from build123d import *

# Parameters (mm, degrees)
BOSS_EXTRUDE1_DEPTH = 2.54
SKETCH2_R           = 1.016
CUT_EXTRUDE1_DEPTH  = 3.54


with BuildPart() as part:
    # Sketch1 → Boss-Extrude1 (new body)
    with BuildSketch(Plane(origin=(0, 0, 0), x_dir=(1, 0, 0), z_dir=(0, 1, 0))):
        with BuildLine():
            Line((0, 0), (10.16, 0))
            ThreePointArc((10.16, 0), (13.97, 3.81), (10.16, 7.62))
            Line((10.16, 7.62), (0, 7.62))
            ThreePointArc((0, 7.62), (-3.81, 3.81), (0, 0))
        make_face()
    extrude(amount=BOSS_EXTRUDE1_DEPTH)

    # Sketch2 → Cut-Extrude1 (cut, through all)
    with BuildSketch(Plane(origin=(0, 2.54, 0), x_dir=(1, 0, 0), z_dir=(0, 1, 0))):
        with Locations((0, 3.81)):
            Circle(SKETCH2_R)
        with Locations((5.08, 3.81)):
            Circle(SKETCH2_R)
        with Locations((10.16, 3.81)):
            Circle(SKETCH2_R)
    extrude(amount=-CUT_EXTRUDE1_DEPTH, mode=Mode.SUBTRACT)


solid = part.part
Design review of the part built by this model. Coordinates are the model's own, in mm. Round coordinates to 2 decimals unless told otherwise and drop trailing zeros. Loops run counter-clockwise (first coordinate to the right, second up) from the corner with the lowest first, then second, coordinate; pieces in that order, holes last. Notation, with made-up numbers: (-1.75, 79.25) -> (47.25, 79.25) arc R23 cw to (47.25, 112.25) -> close; hole circle Ø4 at (-11.75, -33.75). An arc over 180 degrees is marked (long way). Use one line per item in the form item = value. Start each with the question number.
Q1. For pin 1 Ø1 at (x, y) = (-1, 2) entering from -Z; pin 2 Ø2.5 at (x, z) = (5.08, -3.81) entering from +Y, all flat-tipped, find the tip position at first contact; note any pin that passes through.
Q2. Wall thickness on line 1 along X through (y, z) = (0.55, -3.81); line 2 along Z through (x, y) = (0, 1.6); line 3 along X through (y, z) = (1.45, -4): over which ranges is each line inside the solid? List them lowest first. Write a range as [from, to].
Q3. Draft analysis for pull direction Z (two halves, no side actions). For faces 1 (the face through (-3.81, 1.25, -3.89)), 2 (the face through (-0.132, 1.288, -4.817)), 3 (the face through (7, 0, -4)), 4 (the face through (5, 1, -7.62)), state which applies: +Z half, -Z half, draft (parallel to the pull), parting line (faces both ways), or undercut.
Q4. We need section D-D on z = -2.25. Give the boundary of the cut face in (x, y), then the cut area to 3 significant figures.
Q5. We need section B-B on y = 1.9. Give the boundary of the cut face in (x, z).
Q6. We need section C-C on z = -3.81. Give the boundary of the cut face in (x, y).
Q7. We need section A-A on x = 5.08. Give the boundary of the cut face in (y, z), then the cut area to 3 significant figures.
Calculated:
q1.pin_1 = -7.59
q1.pin_2 = 2.54
q2.line_1 = [-3.81, -1.02], [1.02, 4.06], [6.1, 9.14], [11.18, 13.97]
q2.line_2 = [-7.62, -4.83], [-2.79, 0]
q2.line_3 = [-3.81, -1], [1, 4.08], [6.08, 9.16], [11.16, 13.97]
q3.face_1 = parting line
q3.face_2 = undercut
q3.face_3 = draft
q3.face_4 = -Z half
q4.outline = (-3.48, 0) -> (13.64, 0) -> (13.64, 2.54) -> (-3.48, 2.54) -> close
q4.area = 43.5 mm²
q5.outline = (0, -7.62) -> (10.16, -7.62) arc R3.81 ccw to (10.16, 0) -> (0, 0) arc R3.81 ccw to start; hole circle Ø2.03 at (0, -3.81); hole circle Ø2.03 at (5.08, -3.81); hole circle Ø2.03 at (10.16, -3.81)
q6.outline = (-3.81, 0) -> (-1.02, 0) -> (-1.02, 2.54) -> (-3.81, 2.54) -> close; (1.02, 0) -> (4.06, 0) -> (4.06, 2.54) -> (1.02, 2.54) -> close; (6.1, 0) -> (9.14, 0) -> (9.14, 2.54) -> (6.1, 2.54) -> close; (11.18, 0) -> (13.97, 0) -> (13.97, 2.54) -> (11.18, 2.54) -> close
q7.outline = (0, -7.62) -> (2.54, -7.62) -> (2.54, -4.83) -> (0, -4.83) -> close; (0, -2.79) -> (2.54, -2.79) -> (2.54, 0) -> (0, 0) -> close
q7.area = 14.2 mm²
